```python
from build123d import *

# Parameters (mm, degrees)
SKETCH1_R           = 9
BOSS_EXTRUDE1_DEPTH = 3
CUT_EXTRUDE1_DEPTH  = 4
FILLET1_R           = 1


with BuildPart() as part:
    # Sketch1 → Boss-Extrude1 (new body)
    with BuildSketch(Plane(origin=(0, 0, 0), x_dir=(1, 0, 0), z_dir=(0, 1, 0))):
        with BuildLine():
            Line((3.491378029, 30.5), (-3.491378029, 30.5))
            ThreePointArc((-3.491378029, 30.5), (-5.40479519, 30.119397663), (-7.026911935, 29.035533906))
            Line((-7.026911935, 29.035533906), (-29.035533906, 7.026911935))
            ThreePointArc((-29.035533906, 7.026911935), (-30.119397663, 5.40479519), (-30.5, 3.491378029))
            Line((-30.5, 3.491378029), (-30.5, -3.491378029))
            ThreePointArc((-30.5, -3.491378029), (-30.119397663, -5.40479519), (-29.035533906, -7.026911935))
            Line((-29.035533906, -7.026911935), (-7.026911935, -29.035533906))
            ThreePointArc((-7.026911935, -29.035533906), (-5.40479519, -30.119397663), (-3.491378029, -30.5))
            Line((-3.491378029, -30.5), (3.491378029, -30.5))
            ThreePointArc((3.491378029, -30.5), (5.40479519, -30.119397663), (7.026911935, -29.035533906))
            Line((7.026911935, -29.035533906), (21.779928926, -14.282516914))
            ThreePointArc((21.779928926, -14.282516914), (14, 0), (21.779928926, 14.282516914))
            Line((21.779928926, 14.282516914), (7.026911935, 29.035533906))
            ThreePointArc((7.026911935, 29.035533906), (5.40479519, 30.119397663), (3.491378029, 30.5))
        make_face()
        Circle(SKETCH1_R, mode=Mode.SUBTRACT)
    extrude(amount=BOSS_EXTRUDE1_DEPTH)

    # Sketch4 → Cut-Extrude1 (cut, through all)
    with BuildSketch(Plane(origin=(0, 3, 0), x_dir=(1, 0, 0), z_dir=(0, 1, 0))):
        Polygon((-26.25, 7.929437252), (-26.25, 6.129437252), (-24.9, 6.129437252), (-24.9, 4.779437252), (-23.1, 4.779437252), (-23.1, 6.129437252), (-21.75, 6.129437252), (-21.75, 7.929437252), (-23.1, 7.929437252), (-23.1, 9.279437252), (-24.9, 9.279437252), (-24.9, 7.929437252), align=None)
        Polygon((-23.1, -4.779437252), (-24.9, -4.779437252), (-24.9, -6.129437252), (-26.25, -6.129437252), (-26.25, -7.929437252), (-24.9, -7.929437252), (-24.9, -9.279437252), (-23.1, -9.279437252), (-23.1, -7.929437252), (-21.75, -7.929437252), (-21.75, -6.129437252), (-23.1, -6.129437252), align=None)
        Polygon((7.929437252, 23.1), (9.279437252, 23.1), (9.279437252, 24.9), (7.929437252, 24.9), (7.929437252, 26.25), (6.129437252, 26.25), (6.129437252, 24.9), (4.779437252, 24.9), (4.779437252, 23.1), (6.129437252, 23.1), (6.129437252, 21.75), (7.929437252, 21.75), align=None)
        Polygon((26.25, -7.929437252), (26.25, -6.129437252), (24.9, -6.129437252), (24.9, -4.779437252), (23.1, -4.779437252), (23.1, -6.129437252), (21.75, -6.129437252), (21.75, -7.929437252), (23.1, -7.929437252), (23.1, -9.279437252), (24.9, -9.279437252), (24.9, -7.929437252), align=None)
        Polygon((-4.779437252, 24.9), (-6.129437252, 24.9), (-6.129437252, 26.25), (-7.929437252, 26.25), (-7.929437252, 24.9), (-9.279437252, 24.9), (-9.279437252, 23.1), (-7.929437252, 23.1), (-7.929437252, 21.75), (-6.129437252, 21.75), (-6.129437252, 23.1), (-4.779437252, 23.1), align=None)
        Polygon((26.25, 7.929437252), (24.9, 7.929437252), (24.9, 9.279437252), (23.1, 9.279437252), (23.1, 7.929437252), (21.75, 7.929437252), (21.75, 6.129437252), (23.1, 6.129437252), (23.1, 4.779437252), (24.9, 4.779437252), (24.9, 6.129437252), (26.25, 6.129437252), align=None)
        Polygon((-6.129437252, -26.25), (-6.129437252, -24.9), (-4.779437252, -24.9), (-4.779437252, -23.1), (-6.129437252, -23.1), (-6.129437252, -21.75), (-7.929437252, -21.75), (-7.929437252, -23.1), (-9.279437252, -23.1), (-9.279437252, -24.9), (-7.929437252, -24.9), (-7.929437252, -26.25), align=None)
        Polygon((7.929437252, -26.25), (7.929437252, -24.9), (9.279437252, -24.9), (9.279437252, -23.1), (7.929437252, -23.1), (7.929437252, -21.75), (6.129437252, -21.75), (6.129437252, -23.1), (4.779437252, -23.1), (4.779437252, -24.9), (6.129437252, -24.9), (6.129437252, -26.25), align=None)
    extrude(amount=-CUT_EXTRUDE1_DEPTH, mode=Mode.SUBTRACT)

    # Fillet1
    fillet1_edges = [part.edges().sort_by_distance(p)[0] for p in [
        (21.779928926, 1.5, -14.282516914),
        (21.779928926, 1.5, 14.282516914),
    ]]
    fillet(fillet1_edges, radius=FILLET1_R)


solid = part.part
```
Here's how the part is built. I have some questions about the finished solid (model axes, mm). A direction names the side the tool comes from. Round coordinates to 2 decimals unless told otherwise and drop trailing zeros. Order: outer loops, then holes, each group sorted by start corner. A loop starts at its lowest first (then second) coordinate and runs counter-clockwise, first axis right, second up. Notation, with made-up numbers: M 36.25,56.25 L 91.25,56.25 A16 ccw 91.25,77.25 Z; hole C 19.25,7.25 d3. An arc over 180 degrees is marked long. Answer as CSV lines item,"result".
Item 1: Imagine slicing it at D-D on y = 0.55. Give the number of separate pieces and of enclosed holes in the cut face, and give its area (3 significant figures).
From the geometry:
separate pieces,"1"
enclosed holes,"7"
area,"1,810 mm2"
Item 2: Imagine slicing it at B-B on x = 0. List the corners of the cut face in (y, z) for me.
From the geometry:
outline,"M 0,-30.5 L 3,-30.5 L 3,-9 L 0,-9 Z; M 0,9 L 3,9 L 3,30.5 L 0,30.5 Z"
Item 3: Please list where these lines run through material, in increasing order: L1, parallel to X at y = 1.45, z = 0; L2, parallel to Z at x = 0, y = 2.2; L3, parallel to X at y = 0.7, z = -26. Write a range as [from, to].
From the geometry:
L1,"[-30.5, -9], [9, 14]"
L2,"[-30.5, -9], [9, 30.5]"
L3,"[-10.06, -7.93], [-6.13, 6.13], [7.93, 10.06]"
Item 4: We'd pull the mould along X, two halves only. Please class faces 3 (the cylindrical face through (5.43, 1.48, -30.11)), 4 (the flat face through (7, 2, -21.75)), 5 (the flat face through (-11, 3, 0)), 6 (the flat face through (-26, 2, 7.929)): +X half, -X half, draft (parallel to the pull), parting line (faces both ways), or undercut.
From the geometry:
face 3,"+X half"
face 4,"undercut"
face 5,"draft"
face 6,"undercut"
Item 5: Imagine slicing it at A-A on z = 0. List the corners of the cut face in (x, y) for me, and give its area (3 significant figures).
From the geometry:
outline,"M -30.5,0 L -9,0 L -9,3 L -30.5,3 Z; M 9,0 L 14,0 L 14,3 L 9,3 Z"
area,"79.5 mm2"
Item 6: Which directions (+Z, -Z, +X, -X, +Y, -Y) give clear straight access to the entire face, cutting with the end or side of a thin tool? Please do faces 1 (the flat face through (0, 1, 30.5)), 2 (the flat face through (-24, 2, 4.779)).
From the geometry:
face 1,"+Z, +X, -X, +Y, -Y"
face 2,"+Y, -Y"
Item 7: Imagine slicing it at C-C on x = -24. List the corners of the cut face in (y, z) for me, and give its area (3 significant figures).
From the geometry:
outline,"M 0,-12.06 L 3,-12.06 L 3,-9.28 L 0,-9.28 Z; M 0,-4.78 L 3,-4.78 L 3,4.78 L 0,4.78 Z; M 0,9.28 L 3,9.28 L 3,12.06 L 0,12.06 Z"
area,"45.4 mm2"
Item 8: For pin 1 (1.5 mm diameter, centred on y = 1.5, z = -25.5, fed in from +X); pin 2 (1.1 mm diameter, centred on x = -25.5, y = 2, fed in from -Z); pin 3 (1.1 mm diameter, centred on y = 1.5, z = -22.5, fed in from +X), each with a flat end and sliding along its axis, tell me the tip position at first contact or that it passes through.
From the geometry:
pin 1,"x = 11.31"
pin 2,"z = -11.11"
pin 3,"x = 14.11"
